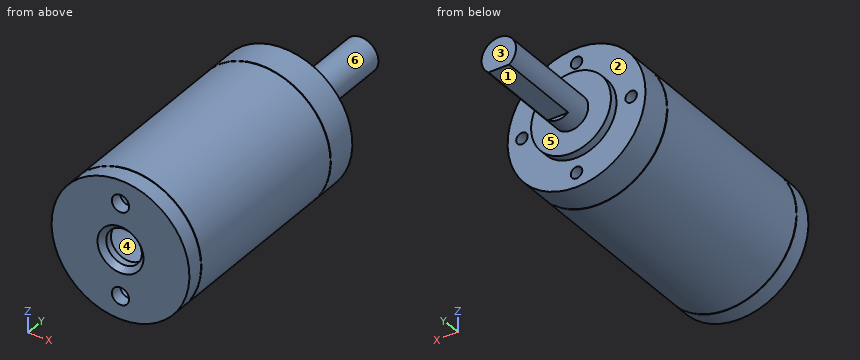
```python
from build123d import *

# Parameters (mm, degrees)
SKETCH_1_R               = 12
EXTRUDE_1_DEPTH          = 41.3
SHELL_6_T                = 2.1
SKETCH_2_R               = 6.95
EXTRUDE_2_DEPTH          = 1.4
SKETCH_3_R               = 3
EXTRUDE_3_DEPTH          = 18.3
CUT_EXTRUDE_1_DEPTH      = 15
SKETCH_5_R               = 3.1
CUT_EXTRUDE_2_DEPTH      = 10
CHAMFER_1_SIZE           = 0.9
SKETCH_7_R               = 1
CUT_EXTRUDE_3_DEPTH      = 10
PATTERN_CIRCULAR_1_COUNT = 4
SKETCH_8_R               = 1.5
CUT_EXTRUDE_4_DEPTH      = 10
PATTERN_CIRCULAR_2_COUNT = 2
SKETCH_10_W              = 1
SKETCH_10_H              = 0.1


with BuildPart() as part:
    # 草图1 → 凸台-拉伸1 (new body)
    with BuildSketch(Plane(origin=(0, 0, 0), x_dir=(1, 0, 0), z_dir=(0, 1, 0))):
        with Locations(Location((0, 0, 0), (0, 0, 90))):
            Circle(SKETCH_1_R)
    extrude(amount=EXTRUDE_1_DEPTH)

    # 抽壳6 (no face opened: a closed hollow body)
    add(offset(amount=-SHELL_6_T, mode=Mode.PRIVATE), mode=Mode.SUBTRACT)

    # 草图2 → 凸台-拉伸2 (add)
    with BuildSketch(Plane(origin=(0, 41.3, 0), x_dir=(1, 0, 0), z_dir=(0, 1, 0))):
        with Locations(Location((0, 0, 0), (0, 0, 270))):
            Circle(SKETCH_2_R)
    extrude(amount=EXTRUDE_2_DEPTH)

    # 草图3 → 凸台-拉伸3 (add)
    with BuildSketch(Plane(origin=(0, 42.7, 0), x_dir=(1, 0, 0), z_dir=(0, 1, 0))):
        with Locations(Location((0, 0, 0), (0, 0, 270))):
            Circle(SKETCH_3_R)
    extrude(amount=EXTRUDE_3_DEPTH)

    # 草图4 → 切除-拉伸1 (cut)
    with BuildSketch(Plane(origin=(0, 61, 0), x_dir=(1, 0, 0), z_dir=(0, 1, 0))):
        Polygon((-4.180388969, 2.4), (5.154958177, 2.4), (-0.718103627, 5.682759436), align=None)
    extrude(amount=-CUT_EXTRUDE_1_DEPTH, mode=Mode.SUBTRACT)

    # 草图5 → 切除-拉伸2 (cut)
    with BuildSketch(Plane.XZ):
        with Locations(Location((0, 0, 0), (0, 0, 270))):
            Circle(SKETCH_5_R)
    extrude(amount=-CUT_EXTRUDE_2_DEPTH, mode=Mode.SUBTRACT)

    # 倒角1
    chamfer_1_edges = [part.edges().sort_by_distance(p)[0] for p in [
        (0, 0, 3.1),
    ]]
    chamfer(chamfer_1_edges, length=CHAMFER_1_SIZE)

    # 草图7 → 切除-拉伸3 (cut)
    with BuildSketch(Plane(origin=(0, 41.3, 0), x_dir=(1, 0, 0), z_dir=(0, 1, 0))):
        with Locations(Location((0, 9.5, 0), (0, 0, 270))):
            Circle(SKETCH_7_R)
    cut_extrude_3 = extrude(amount=-CUT_EXTRUDE_3_DEPTH, mode=Mode.SUBTRACT)

    # 阵列(圆周)1: 切除-拉伸3 ×4 about axis
    pattern_circular_1_axis = Axis((0, 0, 0), (0, 1, 0))
    for i in range(1, PATTERN_CIRCULAR_1_COUNT):
        add(cut_extrude_3.rotate(pattern_circular_1_axis, i * 360 / PATTERN_CIRCULAR_1_COUNT), mode=Mode.SUBTRACT)

    # 草图8 → 切除-拉伸4 (cut)
    with BuildSketch(Plane.XZ):
        with Locations(Location((0, 8, 0), (0, 0, 270))):
            Circle(SKETCH_8_R)
    cut_extrude_4 = extrude(amount=-CUT_EXTRUDE_4_DEPTH, mode=Mode.SUBTRACT)

    # 阵列(圆周)2: 切除-拉伸4 ×2 about axis
    pattern_circular_2_axis = Axis((0, 0, 0), (0, 1, 0))
    for i in range(1, PATTERN_CIRCULAR_2_COUNT):
        add(cut_extrude_4.rotate(pattern_circular_2_axis, i * 360 / PATTERN_CIRCULAR_2_COUNT), mode=Mode.SUBTRACT)

    # 草图10 → 切除-旋转1 (revolve, cut)
    with BuildSketch(Plane.XY, mode=Mode.PRIVATE) as cut_revolve_1_sk:
        with Locations((11.890198227, 35.8)):
            Rectangle(SKETCH_10_W, SKETCH_10_H)
        with Locations((12, 3)):
            Rectangle(SKETCH_10_W, SKETCH_10_H)
    revolve(cut_revolve_1_sk.sketch.rotate(Axis((0, 62.182119541, 0), (0, -1, 0)), 233.130102354), axis=Axis((0, 62.182119541, 0), (0, -1, 0)), mode=Mode.SUBTRACT)


solid = part.part
```
Source: CAD feature listing. Evaluate the final solid. Frame: model axes, mm. Face numbers are marked on the shaded views. A direction names the side the tool comes from. Give positions to 0.01 mm unless a question says otherwise; leave off trailing zeros. Loops run counter-clockwise (first coordinate to the right, second up) from the corner with the lowest first, then second, coordinate; pieces in that order, holes last. Notation, with made-up numbers: (61.5, -22.75) - (68.5, -22.75) arc R13 ccw to (68.5, -13.75) - close; hole circle Ø10 at (-11, 16). An arc over 180 degrees is marked (long way). Use CSV: the item, a comma, the result in double quotes. Start each with the question number.
1. Reachability of the marked faces 1, 2 and 3 from +Z, -Z, +X, -X, +Y, -Y: full face, straight path, thin tool, end or side. Return the list, or none.
2. Section A-A (y = 38.5). Output: boundary loops of the cut face in (x, z).
3. Section B-B (z = 0). Count the separate pieces of the cut face and the enclosed holes in it, then the cut area to 3 significant figures.
4. Ray query, L1, parallel to Y at x = -3, z = -3.25; L2, parallel to Y at x = -8.25, z = 1.25; L3, parallel to X at y = 1.2, z = 0. Return the intervals inside material, ascending.
5. Draft query along X for the marked faces 4, 5 and 6. Return one class per face: +X half, -X half, draft (parallel to the pull), parting line (faces both ways), or undercut.
6. Pin query (flat end, axial travel): pin 1 (2 mm diameter, centred on y = 26, z = 4, fed in from -X); pin 2 (4 mm diameter, centred on x = 9.5, z = -6.5, fed in from +Y); pin 3 (1.8 mm diameter, centred on x = 0.5, y = 54.5, fed in from -Z). Return the tip coordinate at first contact, or that it passes through.
7. Section D-D (y = 26). Output: boundary loops of the cut face in (x, z).
Response:
1,face 1,"-Z, +X, -X, +Y"
1,face 2,"+Y"
1,face 3,"+Z, -Z, +X, -X, +Y"
2,outline,"circle Ø24 at (0, 0); hole (-9.86, -0.93) arc R9.9 ccw to (-0.93, -9.86) arc R1 ccw to (0.93, -9.86) arc R9.9 ccw to (9.86, -0.93) arc R1 ccw to (9.86, 0.93) arc R9.9 ccw to (0.93, 9.86) arc R1 ccw to (-0.93, 9.86) arc R9.9 ccw to (-9.86, 0.93) arc R1 ccw to start"
3,separate pieces,"3"
3,enclosed holes,"0"
3,area,"354 mm²"
4,L1,"0 to 2.1, 39.2 to 42.7"
4,L2,"0 to 2.1, 39.2 to 41.3"
4,L3,"-12 to -3.1, 3.1 to 12"
5,face 4,"undercut"
5,face 5,"draft"
5,face 6,"parting line"
6,pin 1,"x = -11.62"
6,pin 2,"y = 41.3"
6,pin 3,"z = -2.4"
7,outline,"circle Ø24 at (0, 0); hole circle Ø19.8 at (0, 0)"
